Build history of the part. All positions in model axes, mm. Round coordinates to 2 decimals unless told otherwise and drop trailing zeros. Loops run counter-clockwise (first coordinate to the right, second up) from the corner with the lowest first, then second, coordinate; pieces in that order, holes last.
from build123d import *

# Parameters (mm, degrees)
SKETCH1_R           = 2.125
SKETCH1_W           = 19.725
SKETCH1_H           = 4
BOSS_EXTRUDE1_DEPTH = 4


with BuildPart() as part:
    # Sketch1 → Boss-Extrude1 (new body)
    with BuildSketch(Plane(origin=(0, 0, 0), x_dir=(1, 0, 0), z_dir=(0, 1, 0))):
        Polygon((299.8, 24), (299.8, 4), (295.8, 4), (295.8, -16), (299.8, -16), (299.8, -36), (295.8, -36), (295.8, -56), (299.8, -56), (299.8, -76), (275.8, -76), (275.8, -6), (-275.8, -6), (-275.8, -76), (-299.8, -76), (-299.8, -56), (-295.8, -56), (-295.8, -36), (-299.8, -36), (-299.8, -16), (-295.8, -16), (-295.8, 4), (-299.8, 4), (-299.8, 24), align=None)
        with Locations((285.8, -67.5)):
            Circle(SKETCH1_R, mode=Mode.SUBTRACT)
        with Locations((285.8, -54.75)):
            Circle(SKETCH1_R, mode=Mode.SUBTRACT)
        with Locations((-285.8, -54.75)):
            Circle(SKETCH1_R, mode=Mode.SUBTRACT)
        with Locations((-285.8, -67.5)):
            Circle(SKETCH1_R, mode=Mode.SUBTRACT)
        with Locations((0, 2)):
            Rectangle(SKETCH1_W, SKETCH1_H, mode=Mode.SUBTRACT)
        with Locations((39.45, 2)):
            Rectangle(SKETCH1_W, SKETCH1_H, mode=Mode.SUBTRACT)
        with Locations((78.87, 2)):
            Rectangle(SKETCH1_W, SKETCH1_H, mode=Mode.SUBTRACT)
        with Locations((118.29, 2)):
            Rectangle(SKETCH1_W, SKETCH1_H, mode=Mode.SUBTRACT)
        with Locations((157.71, 2)):
            Rectangle(SKETCH1_W, SKETCH1_H, mode=Mode.SUBTRACT)
        with Locations((197.13, 2)):
            Rectangle(SKETCH1_W, SKETCH1_H, mode=Mode.SUBTRACT)
        with Locations((236.55, 2)):
            Rectangle(SKETCH1_W, SKETCH1_H, mode=Mode.SUBTRACT)
        with Locations((275.97, 2)):
            Rectangle(SKETCH1_W, SKETCH1_H, mode=Mode.SUBTRACT)
        with Locations((-275.97, 2)):
            Rectangle(SKETCH1_W, SKETCH1_H, mode=Mode.SUBTRACT)
        with Locations((-236.55, 2)):
            Rectangle(SKETCH1_W, SKETCH1_H, mode=Mode.SUBTRACT)
        with Locations((-197.13, 2)):
            Rectangle(SKETCH1_W, SKETCH1_H, mode=Mode.SUBTRACT)
        with Locations((-157.71, 2)):
            Rectangle(SKETCH1_W, SKETCH1_H, mode=Mode.SUBTRACT)
        with Locations((-118.29, 2)):
            Rectangle(SKETCH1_W, SKETCH1_H, mode=Mode.SUBTRACT)
        with Locations((-78.87, 2)):
            Rectangle(SKETCH1_W, SKETCH1_H, mode=Mode.SUBTRACT)
        with Locations((-39.45, 2)):
            Rectangle(SKETCH1_W, SKETCH1_H, mode=Mode.SUBTRACT)
    extrude(amount=BOSS_EXTRUDE1_DEPTH)


solid = part.part
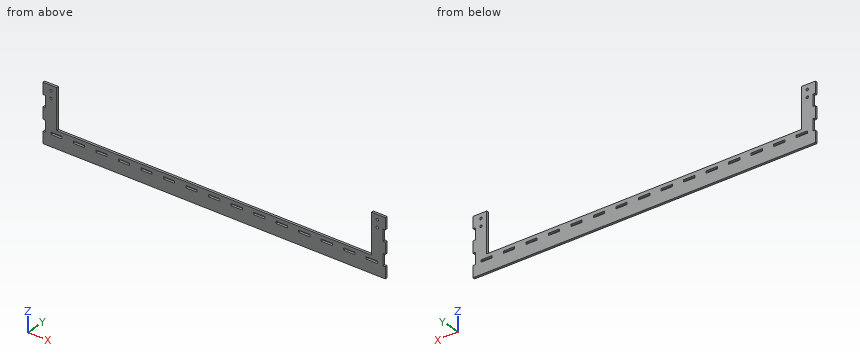
(1) Slice it at C-C on x = -98. List the corners of the cut face in (y, z), plus the area to 3 significant figures.
Responses:
outline: (0, -24) - (4, -24) - (4, 6) - (0, 6) - close
area: 120 mm2
(2) Slice it at B-B on y = 1.3. Count the separate pieces of the cut face and the enclosed holes in it, plus the area to 3 significant figures.
Responses:
separate pieces: 1
enclosed holes: 19
area: 19,800 mm2
(3) Slice it at A-A on z = 24. List the corners of the cut face in (x, y), plus the area to 3 significant figures.
Responses:
outline: (-299.8, 0) - (-275.8, 0) - (-275.8, 4) - (-299.8, 4) - close; (275.8, 0) - (299.8, 0) - (299.8, 4) - (275.8, 4) - close
area: 192 mm2
(4) Pin check, flat tips, straight feed: P1, Ø1.2, axis at x = 198.5, y = 2.5, coming from the +Z side; P2, Ø1, axis at x = -86, z = 8, coming from the -Y side; P3, Ø1.2, axis at y = 2.5, z = -1.5, coming from the +X side. Stop position of each tip, or through.
Responses:
P1: stops at z = 6
P2: passes through
P3: stops at x = 295.8
(5) Probe line 1 (X direction, y = 2.7, z = 67.5) (3 decimals); line 2 (X direction, y = 1.95, z = 54.75) (3 decimals); line 3 (Z direction, x = 285.8, y = 1.8) (3 decimals). List the from-to ranges inside material, lowest first.
Responses:
line 1: x = -299.8 to -287.925, -283.675 to -275.8, 275.8 to 283.675, 287.925 to 299.8
line 2: x = -295.8 to -287.925, -283.675 to -275.8, 275.8 to 283.675, 287.925 to 295.8
line 3: z = -24 to -4, 0 to 52.625, 56.875 to 65.375, 69.625 to 76
